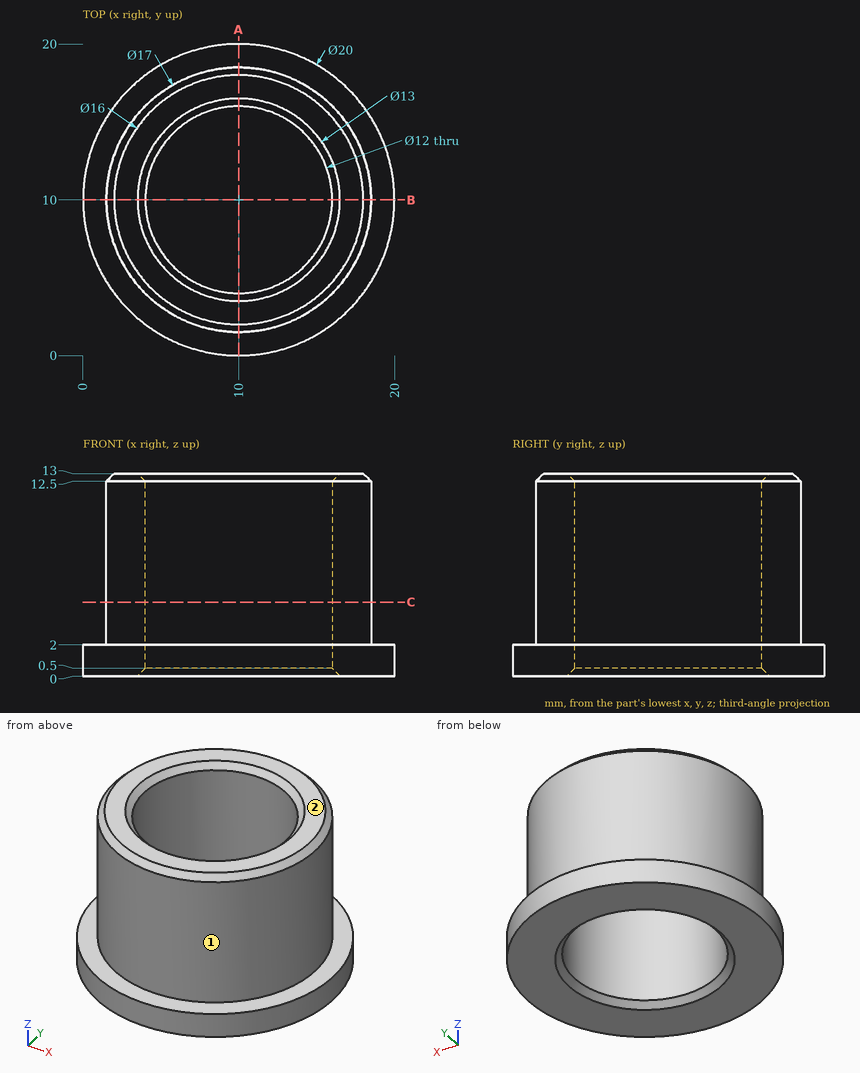
Design review of the part shown in the three views and the two pictorial views. Dimensions are in mm from the part's minimum x, y and z. A direction names the side the tool comes from. Give positions to 0.01 mm unless a question says otherwise; leave off trailing zeros. Loops run counter-clockwise (first coordinate to the right, second up) from the corner with the lowest first, then second, coordinate; pieces in that order, holes last. Notation, with made-up numbers: (62, 1) -> (120, 1) arc R15 cw to (120, 16) -> close; hole circle Ø8 at (-11, -36.5). An arc over 180 degrees is marked (long way). Put each result on its own line as item: value. Start each with the question number.
1. For the marked faces 1 and 2, list the 3-axis set-ups (+Z, -Z, +X, -X, +Y, -Y) from which the entire face can be reached by the end or side of a thin tool; tool diameter is ignored.
2. Wall thickness on probe 1 along Y at (x, z) = (10, 7.25); probe 2 along Y at (x, z) = (15, 10.5); probe 3 along Z at (x, y) = (19, 10.75): over which ranges is each line inside the solid? List them lowest first.
3. Clearance check with flat-ended pins moving along their axes: P1, Ø1, axis at x = 15, z = 11, coming from the +Y side; P2, Ø4, axis at y = 8.5, z = 5.5, coming from the +X side; P3, Ø1.5, axis at x = 15.5, y = 9, coming from the +Z side; P4, Ø12, axis at x = 7.5, y = 11, coming from the +Z side. State where each tip first meets the part, or that it passes through.
4. We need section A-A on x = 10. State the section outline as (y, z) points.
5. We need section C-C on z = 4.75. State the section outline as (x, y) points, then the cut area to 3 significant figures.
Determined:
1. face 1: +Z
1. face 2: +Z, +X, -X, +Y, -Y
2. probe 1: 1.5 to 4, 16 to 18.5
2. probe 2: 3.13 to 6.68, 13.32 to 16.87
2. probe 3: 0 to 2
3. P1: y = 17.21
3. P2: x = 18.5
3. P3: z = 12.84
3. P4: z = 13
4. outline: (0, 0) -> (3.5, 0) -> (4, 0.5) -> (4, 12.5) -> (3.5, 13) -> (2, 13) -> (1.5, 12.5) -> (1.5, 2) -> (0, 2) -> close; (16, 0.5) -> (16.5, 0) -> (20, 0) -> (20, 2) -> (18.5, 2) -> (18.5, 12.5) -> (18, 13) -> (16.5, 13) -> (16, 12.5) -> close
5. outline: circle Ø17 at (10, 10); hole circle Ø12 at (10, 10)
5. area: 114 mm^2
